from build123d import *

# Parameters (mm, degrees)
BOSS_EXTRUDE1_DEPTH = 35
SKETCH3_R           = 3.0015
CUT_EXTRUDE1_DEPTH  = 58.606470928
SKETCH3_5_R         = 9
CUT_EXTRUDE2_DEPTH  = 2
SKETCH4_R           = 1.7
CUT_EXTRUDE3_DEPTH  = 58.272989631
CHAMFER1_SIZE       = 5


with BuildPart() as part:
    # Sketch1 → Boss-Extrude1 (new body)
    with BuildSketch(Plane(origin=(0, 0, 0), x_dir=(0, 0, -1), z_dir=(1, 0, 0))):
        Polygon((0, 35), (0, 0), (40, 0), (40, 12.785016481), (11.186889421, 12.785016481), (11.186889421, 35), align=None)
    extrude(amount=BOSS_EXTRUDE1_DEPTH)

    # Sketch3 → Cut-Extrude1 (cut, through all)
    with BuildSketch(Plane(origin=(0, 12.785016481, 0), x_dir=(1, 0, 0), z_dir=(0, 1, 0))):
        with Locations(Location((17.5, 25.59344471, 0), (0, 0, 270))):
            Circle(SKETCH3_R)
    extrude(amount=-CUT_EXTRUDE1_DEPTH, mode=Mode.SUBTRACT)

    # Sketch3<5> → Cut-Extrude2 (cut)
    with BuildSketch(Plane(origin=(0, 12.785016481, 0), x_dir=(1, 0, 0), z_dir=(0, 1, 0))):
        with Locations(Location((17.5, 25.59344471, 0), (0, 0, 270))):
            Circle(SKETCH3_5_R)
    extrude(amount=-CUT_EXTRUDE2_DEPTH, mode=Mode.SUBTRACT)

    # Sketch4 → Cut-Extrude3 (cut, through all)
    with BuildSketch(Plane(origin=(0, 0, -11.186889421), x_dir=(-1, 0, 0), z_dir=(0, 0, -1))):
        with Locations((-31.00681869, 31.616501478)):
            Circle(SKETCH4_R)
        with Locations((-31.00681869, 17.332786674)):
            Circle(SKETCH4_R)
        with Locations((-4.00681869, 17.332786674)):
            Circle(SKETCH4_R)
        with Locations((-4.00681869, 31.616501478)):
            Circle(SKETCH4_R)
    extrude(amount=-CUT_EXTRUDE3_DEPTH, mode=Mode.SUBTRACT)

    # Chamfer1
    # the kernel refuses this chamfer: 5 mm, written as the material it adds along each edge
    with BuildSketch(Plane(origin=(0, 12.785016481, -11.186889421), x_dir=(0, 0.9996219169112968, 0.02749587661058631), z_dir=(1, 0, 0))) as chamfer1_piece_1_section:
        Polygon((CHAMFER1_SIZE * 0.999621916911, -CHAMFER1_SIZE * 0.0274958766106), (-CHAMFER1_SIZE * 0.0274958766106, -CHAMFER1_SIZE * 0.999621916911), (0, 0), align=None)
    chamfer1_piece_1 = extrude(amount=35, mode=Mode.PRIVATE)
    chamfer1_piece_1 = chamfer1_piece_1 - Plane(origin=(31.00681869, 17.332786674, -12.868450171), x_dir=(-1, 0, 0), z_dir=(0, 0, -1)) * Cylinder(1.7, 90, mode=Mode.PRIVATE)
    chamfer1_piece_1 = chamfer1_piece_1 - Plane(origin=(4.00681869, 17.332786674, -12.868450171), x_dir=(-1, 0, 0), z_dir=(0, 0, -1)) * Cylinder(1.7, 90, mode=Mode.PRIVATE)
    add(chamfer1_piece_1)


solid = part.part
Read the model definition and answer for the solid it produces. Units are mm, in the model's axes. A direction names the side the tool comes from. Give positions to 0.01 mm unless a question says otherwise; leave off trailing zeros. Write each loop counter-clockwise with the first axis right and the second up, starting at its lowest first coordinate (ties: lowest second). Pieces come first, ordered by that corner, then holes. Notation, with made-up numbers: (66, 21) -> (85, 21) arc R24 cw to (85, 31) -> close; hole circle Ø3 at (4, 65). An arc over 180 degrees is marked (long way). Answer as a JSON object with one key per item and string values. Group by question number.
1) A tool of negligible diameter and unlimited length cuts with its end or side. For faces 5 (the cylindrical face through (2.909, 16.035, -5.303)), 6 (the cylindrical face through (20.2, 11.8, -17.01)), 7 (the flat face through (17, 12.785, -36)), from which of +Z, -Z, +X, -X, +Y, -Y can it reach the whole face along a straight path? Write none if from no direction.
2) Find section C-C (z = -10.5). Write down the section's boundary in (x, y).
3) Find section A-A (x = 17.5). Write down the section's boundary in (y, z), and give its area (3 significant figures).
4) Each of these flat-tipped pins is pushed along its axis until it touches: P1, Ø4.5, axis at x = 4.01, y = 17.33, coming from the -Z side; P2, Ø20, axis at x = 17.5, z = -24.5, coming from the +Y side; P3, Ø6, axis at x = 10.5, y = 28, coming from the -Z side. Where does it stop, or does it pass through?
5) Find section B-B (z = -27). Write down the section's boundary in (x, y).
6) The mould has two halves that part along X. Classify faces 1 (the flat face through (20, 10.785, -28)), 2 (the flat face through (17, 6, -40)), 3 (the flat face through (0, 13.6, -15)), 4 (the cylindrical face through (29.909, 16.035, -5.303)): +X half, -X half, draft (parallel to the pull), parting line (faces both ways), or undercut.
7) Consider L1, parallel to Y at x = 28, z = -31.5; L2, parallel to Z at x = 2, y = 34; L3, parallel to Z at x = 17, y = 12. Determine where each line is inside the solid, lowest interval first. Write a range as from..to.
8) Find section D-D (x = 31). Write down the section's boundary in (y, z), and give its area (3 significant figures).
Values follow:
{
 "1": {"face 5": "+Z, -Z", "face 6": "+Y", "face 7": "-Z, +X, -X, +Y"},
 "2": {"outline": "(0, 0) -> (35, 0) -> (35, 35) -> (0, 35) -> close; hole circle Ø3.4 at (4.01, 17.33); hole circle Ø3.4 at (4.01, 31.62); hole circle Ø3.4 at (31.01, 17.33); hole circle Ø3.4 at (31.01, 31.62)"},
 "3": {"outline": "(0, -40) -> (12.79, -40) -> (12.79, -34.59) -> (10.79, -34.59) -> (10.79, -28.59) -> (0, -28.59) -> close; (0, -22.59) -> (10.79, -22.59) -> (10.79, -16.59) -> (12.79, -16.59) -> (12.79, -16.19) -> (17.79, -11.19) -> (35, -11.19) -> (35, 0) -> (0, 0) -> close", "area": "672 mm2"},
 "4": {"P1": "stops at z = -13.89", "P2": "stops at y = 14.47", "P3": "stops at z = -11.19"},
 "5": {"outline": "(0, 0) -> (14.85, 0) -> (14.85, 10.79) -> (8.61, 10.79) -> (8.61, 12.79) -> (0, 12.79) -> close; (20.15, 0) -> (35, 0) -> (35, 12.79) -> (26.39, 12.79) -> (26.39, 10.79) -> (20.15, 10.79) -> close"},
 "6": {"face 1": "undercut", "face 2": "draft", "face 3": "-X half", "face 4": "undercut"},
 "7": {"L1": "y = 0..12.79", "L2": "z = -11.19..0", "L3": "z = -40..-34.58, -16.61..0"},
 "8": {"outline": "(0, -40) -> (12.79, -40) -> (12.79, -16.19) -> (15.63, -13.34) -> (15.63, 0) -> (0, 0) -> close; (19.03, -11.19) -> (29.92, -11.19) -> (29.92, 0) -> (19.03, 0) -> close; (33.32, -11.19) -> (35, -11.19) -> (35, 0) -> (33.32, 0) -> close", "area": "694 mm2"}
}
